from build123d import *

# Parameters (mm, degrees)
SKETCH1_W           = 185
SKETCH1_H           = 35
SKETCH1_R           = 4.125
BOSS_EXTRUDE1_DEPTH = 3
SKETCH2_R           = 2
CUT_EXTRUDE1_DEPTH  = 4


with BuildPart() as part:
    # Sketch1 → Boss-Extrude1 (new body)
    with BuildSketch(Plane(origin=(0, 0, 0), x_dir=(1, 0, 0), z_dir=(0, 1, 0))):
        Rectangle(SKETCH1_W, SKETCH1_H)
        with Locations((80, 0)):
            Circle(SKETCH1_R, mode=Mode.SUBTRACT)
    extrude(amount=BOSS_EXTRUDE1_DEPTH)

    # Sketch2 → Cut-Extrude1 (cut, through all)
    with BuildSketch(Plane(origin=(0, 3, 0), x_dir=(1, 0, 0), z_dir=(0, 1, 0))):
        with Locations((-87, -0.5)):
            Circle(SKETCH2_R)
        with Locations((-52, -0.5)):
            Circle(SKETCH2_R)
    extrude(amount=-CUT_EXTRUDE1_DEPTH, mode=Mode.SUBTRACT)


solid = part.part
Work out the finished part from the listing and answer in its coordinate system (mm). Round coordinates to 2 decimals unless told otherwise and drop trailing zeros. Order: outer loops, then holes, each group sorted by start corner. A loop starts at its lowest first (then second) coordinate and runs counter-clockwise, first axis right, second up. Notation, with made-up numbers: M 11,-25.75 L 59,-25.75 A13 ccw 59,-19.75 Z; hole C 22,77.5 d1. An arc over 180 degrees is marked long. Put each result on its own line as item: value. Start each with the question number.
Q1. A flat-ended cylindrical pin translates along its axis: pin 1 (2.5 mm diameter, centred on x = -52, z = 0.5, fed in from -Y). Find the tip coordinate at first contact, or state that the pin passes through.
Q2. Section A-A, the plane x = 80 is taken. Write down the section's boundary in (y, z) (3 decimals).
Q3. Section B-B, the plane x = -52 is taken. Write down the section's boundary in (y, z).
Q4. For a pull along X with two mould halves and no side action, classify faces 1 (the flat face through (92.5, 1, 0)), 2 (the cylindrical face through (-53.998, 1.521, 0.412)), 3 (the flat face through (-1, 1, 17.5)), 4 (the cylindrical face through (-85.092, 1.521, -0.101)) as pulls with the +X half, pulls with the -X half, needs draft (parallel to the pull), parting line crosses it, or undercut.
Q5. Straight lines are drawn through the part: L1, parallel to X at y = 1.6, z = 0.5; L2, parallel to Z at x = -52, y = 1.3; L3, parallel to Z at x = 80, y = 2 (3 decimals). For each, find the intervals that lie inside material, in ascending order. Write a range as [from, to].
Findings below:
1. pin 1: passes through
2. outline: M 0,-17.5 L 3,-17.5 L 3,-4.125 L 0,-4.125 Z; M 0,4.125 L 3,4.125 L 3,17.5 L 0,17.5 Z
3. outline: M 0,-17.5 L 3,-17.5 L 3,-1.5 L 0,-1.5 Z; M 0,2.5 L 3,2.5 L 3,17.5 L 0,17.5 Z
4. face 1: pulls with the +X half
4. face 2: undercut
4. face 3: needs draft
4. face 4: undercut
5. L1: x = [-92.5, -89], [-85, -54], [-50, 75.91], [84.09, 92.5]
5. L2: z = [-17.5, -1.5], [2.5, 17.5]
5. L3: z = [-17.5, -4.125], [4.125, 17.5]
